from build123d import *

# Parameters (mm, degrees)
CROQUIS1_W              = 16.5
CROQUIS1_H              = 17
CROQUIS1_R              = 1.5
CROQUIS1_W_2            = 5
SALIENTE_EXTRUIR1_DEPTH = 2
SALIENTE_EXTRUIR2_DEPTH = 2
CROQUIS4_W              = 7
CROQUIS4_H              = 2
SALIENTE_EXTRUIR3_DEPTH = 6
CROQUIS7_W              = 42.522469992
CROQUIS7_H              = 40
SALIENTE_EXTRUIR5_DEPTH = 2
CORTAR_EXTRUIR1_REACH   = 43.113
CROQUIS8_W              = 5
CROQUIS8_H              = 5
REDONDEO1_R             = 5
REDONDEO2_R             = 2
CORTAR_EXTRUIR3_REACH   = 43.113
CROQUIS12_W             = 3
CROQUIS12_H             = 8
REDONDEO3_R             = 1


with BuildPart() as part:
    # Croquis1 → Saliente-Extruir1 (new body)
    # profile 1 of 3: a face of its own
    with BuildSketch(Plane(origin=(0, 0, 0), x_dir=(1, 0, 0), z_dir=(0, 1, 0))):
        with Locations((-26.25, 0)):
            Rectangle(CROQUIS1_W, CROQUIS1_H)
    # profile 2 of 3: a face of its own
    with BuildSketch(Plane(origin=(0, 0, 0), x_dir=(1, 0, 0), z_dir=(0, 1, 0))):
        Polygon((13, -13), (-13, -13), (-13, -8.5), (-18, -8.5), (-18, -18), (18, -18), (18, 18), (-18, 18), (-18, 8.5), (-13, 8.5), (-13, 13), (13, 13), align=None)
        with Locations(Location((-15.25, -15.25, 0), (0, 0, 270))):
            Circle(CROQUIS1_R, mode=Mode.SUBTRACT)
        with Locations(Location((15.25, -15.25, 0), (0, 0, 270))):
            Circle(CROQUIS1_R, mode=Mode.SUBTRACT)
        with Locations(Location((-15.25, 15.25, 0), (0, 0, 270))):
            Circle(CROQUIS1_R, mode=Mode.SUBTRACT)
        with Locations(Location((15.25, 15.25, 0), (0, 0, 270))):
            Circle(CROQUIS1_R, mode=Mode.SUBTRACT)
    # profile 3 of 3: a face of its own
    with BuildSketch(Plane(origin=(0, 0, 0), x_dir=(1, 0, 0), z_dir=(0, 1, 0))):
        with Locations((-15.5, 0)):
            Rectangle(CROQUIS1_W_2, CROQUIS1_H)
    extrude(amount=SALIENTE_EXTRUIR1_DEPTH)

    # Croquis2 → Saliente-Extruir2 (add)
    with BuildSketch(Plane(origin=(0, 2, 0), x_dir=(1, 0, 0), z_dir=(0, 1, 0))):
        Polygon((18, 18), (18, 20), (-22, 20), (-22, 8.5), (-18, 8.5), (-18, 18), align=None)
        Polygon((18, -20), (18, -18), (-18, -18), (-18, -8.5), (-22, -8.5), (-22, -20), align=None)
    extrude(amount=-SALIENTE_EXTRUIR2_DEPTH)

    # Croquis4 → Saliente-Extruir3 (add)
    with BuildSketch(Plane(origin=(0, 2, 0), x_dir=(1, 0, 0), z_dir=(0, 1, 0))):
        with Locations((14.5, -19)):
            Rectangle(CROQUIS4_W, CROQUIS4_H)
        with Locations((14.5, 19)):
            Rectangle(CROQUIS4_W, CROQUIS4_H)
    extrude(amount=SALIENTE_EXTRUIR3_DEPTH)

    # Croquis7 → Saliente-Extruir5 (add)
    with BuildSketch(Plane(origin=(0, 8, 0), x_dir=(1, 0, 0), z_dir=(0, 1, 0))):
        with Locations((-3.261234996, 0)):
            Rectangle(CROQUIS7_W, CROQUIS7_H)
    extrude(amount=SALIENTE_EXTRUIR5_DEPTH)

    # Croquis8 → Cortar-Extruir1 (cut, up to next)
    with BuildSketch(Plane(origin=(0, 10, 0), x_dir=(1, 0, 0), z_dir=(0, 1, 0)), mode=Mode.PRIVATE) as cortar_extruir1_sk1:
        with Locations((15.5, -15.5)):
            Rectangle(CROQUIS8_W, CROQUIS8_H)
    cortar_extruir1_tool1 = extrude(cortar_extruir1_sk1.sketch, amount=-CORTAR_EXTRUIR1_REACH, mode=Mode.PRIVATE) & part.part
    # Croquis8 → Cortar-Extruir1 (cut, up to next)
    with BuildSketch(Plane(origin=(0, 10, 0), x_dir=(1, 0, 0), z_dir=(0, 1, 0)), mode=Mode.PRIVATE) as cortar_extruir1_sk2:
        with Locations((15.5, 15.5)):
            Rectangle(CROQUIS8_W, CROQUIS8_H)
    cortar_extruir1_tool2 = extrude(cortar_extruir1_sk2.sketch, amount=-CORTAR_EXTRUIR1_REACH, mode=Mode.PRIVATE) & part.part
    # Croquis8 → Cortar-Extruir1 (cut, up to next)
    with BuildSketch(Plane(origin=(0, 10, 0), x_dir=(1, 0, 0), z_dir=(0, 1, 0)), mode=Mode.PRIVATE) as cortar_extruir1_sk3:
        with Locations((-15.5, 15.5)):
            Rectangle(CROQUIS8_W, CROQUIS8_H)
    cortar_extruir1_tool3 = extrude(cortar_extruir1_sk3.sketch, amount=-CORTAR_EXTRUIR1_REACH, mode=Mode.PRIVATE) & part.part
    # Croquis8 → Cortar-Extruir1 (cut, up to next)
    with BuildSketch(Plane(origin=(0, 10, 0), x_dir=(1, 0, 0), z_dir=(0, 1, 0)), mode=Mode.PRIVATE) as cortar_extruir1_sk4:
        with Locations((-15.5, -15.5)):
            Rectangle(CROQUIS8_W, CROQUIS8_H)
    cortar_extruir1_tool4 = extrude(cortar_extruir1_sk4.sketch, amount=-CORTAR_EXTRUIR1_REACH, mode=Mode.PRIVATE) & part.part
    add(cortar_extruir1_tool1.solids().sort_by_distance((15.5, 10, 15.5))[0], mode=Mode.SUBTRACT)
    add(cortar_extruir1_tool2.solids().sort_by_distance((15.5, 10, -15.5))[0], mode=Mode.SUBTRACT)
    add(cortar_extruir1_tool3.solids().sort_by_distance((-15.5, 10, -15.5))[0], mode=Mode.SUBTRACT)
    add(cortar_extruir1_tool4.solids().sort_by_distance((-15.5, 10, 15.5))[0], mode=Mode.SUBTRACT)

    # Redondeo1
    redondeo1_edges = [part.edges().sort_by_distance(p)[0] for p in [
        (-13, 1, 13),
        (13, 1, 13),
        (13, 1, -13),
        (-13, 1, -13),
    ]]
    fillet(redondeo1_edges, radius=REDONDEO1_R)

    # Redondeo2
    redondeo2_edges = [part.edges().sort_by_distance(p)[0] for p in [
        (-34.5, 1, 8.5),
        (-34.5, 1, -8.5),
    ]]
    fillet(redondeo2_edges, radius=REDONDEO2_R)

    # Croquis12 → Cortar-Extruir3 (cut, up to next)
    with BuildSketch(Plane(origin=(0, 10, 0), x_dir=(1, 0, 0), z_dir=(0, 1, 0)), mode=Mode.PRIVATE) as cortar_extruir3_sk1:
        with Locations((-21.5, 0)):
            Rectangle(CROQUIS12_W, CROQUIS12_H)
    cortar_extruir3_tool1 = extrude(cortar_extruir3_sk1.sketch, amount=-CORTAR_EXTRUIR3_REACH, mode=Mode.PRIVATE) & part.part
    add(cortar_extruir3_tool1.solids().sort_by_distance((-21.5, 10, 0))[0], mode=Mode.SUBTRACT)

    # Redondeo3
    redondeo3_edges = [part.edges().sort_by_distance(p)[0] for p in [
        (-24.522469992, 9, -20),
        (-24.522469992, 9, 20),
        (-18, 9, 13),
        (-18, 9, 18),
        (-13, 9, 18),
        (-13, 9, 13),
        (-18, 9, -18),
        (-18, 9, -13),
        (-13, 9, -13),
        (-13, 9, -18),
        (18, 9, -13),
        (13, 9, -18),
        (13, 9, -13),
        (13, 9, 13),
        (13, 9, 18),
        (18, 9, 13),
        (-22, 1, -8.5),
        (18, 5, -20),
        (-22, 1, -20),
        (18, 5, 20),
        (-22, 1, 8.5),
        (-22, 1, 20),
        (18, 6, 18),
        (18, 6, -18),
    ]]
    fillet(redondeo3_edges, radius=REDONDEO3_R - 0.0001)  # a hair under: the kernel refuses the full size


solid = part.part
For this review, take the finished solid that the model builds, in its own axes (mm). A direction names the side the tool comes from. Give positions to 0.01 mm unless a question says otherwise; leave off trailing zeros. Loops run counter-clockwise (first coordinate to the right, second up) from the corner with the lowest first, then second, coordinate; pieces in that order, holes last.
Item 1: Take a section at D-D, the plane x = 15.25. State the section outline as (y, z) points, and give its area (3 significant figures).
Item 2: Draft analysis for pull direction Z (two halves, no side actions). For faces 4 (the flat face through (-24.522, 9, 0)), 5 (the flat face through (14, 6, -18)), 6 (the flat face through (1, 8.3, 20)), state which applies: +Z half, -Z half, draft (parallel to the pull), parting line (faces both ways), or undercut.
Item 3: Insertion check: pin 1 (1.6 mm diameter, centred on y = 1.5, z = -12, fed in from -X); pin 2 (5 mm diameter, centred on x = -23, y = 1, fed in from -Z); pin 3 (1 mm diameter, centred on x = -29, y = 0.5, fed in from +Z); pin 4 (2 mm diameter, centred on y = 9, z = 8.5, fed in from -X). Each pin has a flat end and moves straight along its axis. Give the tip position at first contact, or say it passes through.
Item 4: Take a section at B-B, the plane x = -15.25. State the section outline as (y, z) points.
Item 5: Tool access review of faces 1 (the flat face through (-22, 1, 14)), 2 (the flat face through (-16, 9, 13)), 3 (the flat face through (0, 1, -13)): name each direction out of +Z, -Z, +X, -X, +Y, -Y from which nothing blocks a thin tool from reaching the whole face with its end or side.
Item 6: For line 1 along X through (y, z) = (1, -15.25); line 2 along X through (y, z) = (1.75, -0.5); line 3 along Y through (x, z) = (-3.5, 17.5), list the stretches that pass through material, from the lowest coordinate up.
Item 7: Take a section at A-A, the plane z = 15.25. State the section outline as (x, y) points.
Calculated:
1. outline: (0, -20) - (10, -20) - (10, -18) - (2, -18) - (2, -16.75) - (0, -16.75) - close; (0, -13.75) - (2, -13.75) - (2, 13.75) - (0, 13.75) - close; (0, 16.75) - (2, 16.75) - (2, 18) - (10, 18) - (10, 20) - (0, 20) - close; (8, -13) - (10, -13) - (10, 13) - (8, 13) - close
1. area: 152 mm2
2. face 4: draft
2. face 5: undercut
2. face 6: +Z half
3. pin 1: stops at x = -22
3. pin 2: stops at z = -20
3. pin 3: stops at z = 8.5
3. pin 4: stops at x = -24.52
4. outline: (0, -20) - (2, -20) - (2, -16.75) - (0, -16.75) - close; (0, -13.75) - (2, -13.75) - (2, 13.75) - (0, 13.75) - close; (0, 16.75) - (2, 16.75) - (2, 20) - (0, 20) - close; (8, -20) - (10, -20) - (10, -18) - (8, -18) - close; (8, -13) - (10, -13) - (10, 13) - (8, 13) - close; (8, 18) - (10, 18) - (10, 20) - (8, 20) - close
5. face 1: +Z, -X, -Y
5. face 2: +Y
5. face 3: -Y
6. line 1: x = -22 to -16.75, -13.75 to 13.75, 16.75 to 18
6. line 2: x = -34.5 to -13, 13 to 18
6. line 3: y = 0 to 2, 8 to 10
7. outline: (-24.52, 8) - (-18, 8) - (-18, 10) - (-24.52, 10) - close; (-22, 0) - (-16.75, 0) - (-16.75, 2) - (-22, 2) - close; (-13.75, 0) - (13.75, 0) - (13.75, 2) - (-13.75, 2) - close; (-13, 8) - (13, 8) - (13, 10) - (-13, 10) - close; (16.75, 0) - (18, 0) - (18, 2) - (16.75, 2) - close
